```python
from build123d import *

# Parameters (mm, degrees)
SKETCH_1_R               = 3.2
EXTRUDE_1_DEPTH          = 5
CUT_EXTRUDE_1_DEPTH      = 5
CUT_EXTRUDE_1_DEPTH_BACK = 5
SKETCH_2_R               = 1.5


with BuildPart() as part:
    # Sketch 1 → Extrude 1 (new body)
    with BuildSketch(Plane.XY):
        with BuildLine():
            Line((-3.31662479, -5), (-8.660254038, -5))
            Line((-8.660254038, -5), (-8.660254038, 5))
            Line((-8.660254038, 5), (-4, 5))
            Line((-4, 5), (-4, 9.16515139))
            Line((-4, 9.16515139), (3, 9.16515139))
            Line((3, 9.16515139), (3, 5))
            Line((3, 5), (6.81662479, 5))
            Line((6.81662479, 5), (6.81662479, -5))
            Line((6.81662479, -5), (3.31662479, -5))
            ThreePointArc((3.31662479, -5), (0, -6), (-3.31662479, -5))
        make_face()
        Circle(SKETCH_1_R, mode=Mode.SUBTRACT)
    extrude(amount=EXTRUDE_1_DEPTH)

    # Sketch 2 → Cut-Extrude 1 (cut, two sides: drawn at the far end of the back side and taken through both)
    with BuildSketch(Plane.XZ.offset(5).offset(-CUT_EXTRUDE_1_DEPTH_BACK)):
        with Locations(Location((0, 2.9, 0), (0, 0, 90))):
            Circle(SKETCH_2_R)
    extrude(amount=CUT_EXTRUDE_1_DEPTH + CUT_EXTRUDE_1_DEPTH_BACK, mode=Mode.SUBTRACT)


solid = part.part
```
The listing builds one solid part. Answer for the finished solid, in the listing's coordinates (mm). A direction names the side the tool comes from. Give positions to 0.01 mm unless a question says otherwise; leave off trailing zeros. Order: outer loops, then holes, each group sorted by start corner. A loop starts at its lowest first (then second) coordinate and runs counter-clockwise, first axis right, second up. Notation, with made-up numbers: (37, 40) - (51, 40) arc R24 cw to (51, 73) - close; hole circle Ø3 at (71, 85). An arc over 180 degrees is marked (long way). Use one line per item in the form item = value. Start each with the question number.
(1) The mould has two halves that part along X. Classify faces 1 (the cylindrical face through (-0.45, -4.39, 4.33)), 2 (the flat face through (-6, -5, 2)), 3 (the flat face through (-4, 7, 2)): released by +X, released by -X, zero draft, split by the parting line, or undercut.
(2) A cutting plane is placed at D-D, the plane x = -2. Write down the section's boundary in (y, z).
(3) For faces 4 (the flat face through (-6, 5, 2)), 5 (the flat face through (5, -5, 2)), 6 (the flat face through (5, 5, 2)), determine the directions among +Z, -Z, +X, -X, +Y, -Y from which every point of the face is accessible in a straight line to the end or side of a thin tool.
(4) A cutting plane is placed at B-B, the plane x = 0. Write down the section's boundary in (y, z).
(5) Consider line 1 (X direction, y = -4.8, z = 2.9); line 2 (Y direction, x = -5, z = 1.5); line 3 (X direction, y = 5.25, z = 2.6). Determine where each line is inside the solid, lowest interval first. Write a range as from..to.
(6) Flat-ended cylindrical pins translate along their axes: pin 1 Ø3 at (x, z) = (-2.5, 1) entering from -Y; pin 2 Ø1.4 at (x, z) = (-6.5, 2) entering from +Y; pin 3 Ø1.2 at (y, z) = (7, 3.5) entering from -X. Find the tip coordinate at first contact, or state that the pin passes through.
(7) A cutting plane is placed at C-C, the plane z = 0.85. Write down the section's boundary in (x, y), then the cut area to 3 significant figures.
(8) A cutting plane is placed at A-A, the plane y = 0. Write down the section's boundary in (x, z).
Ans:
q1.face_1 = undercut
q1.face_2 = zero draft
q1.face_3 = released by -X
q2.outline = (-5.66, 0) - (-2.5, 0) - (-2.5, 5) - (-5.66, 5) - close; (2.5, 0) - (9.17, 0) - (9.17, 5) - (2.5, 5) - close
q3.face_4 = +Z, -Z, -X, +Y
q3.face_5 = +Z, -Z, +X, -Y
q3.face_6 = +Z, -Z, +X, +Y
q4.outline = (-6, 0) - (-3.2, 0) - (-3.2, 1.4) - (-6, 1.4) - close; (-6, 4.4) - (-3.2, 4.4) - (-3.2, 5) - (-6, 5) - close; (3.2, 0) - (9.17, 0) - (9.17, 5) - (3.2, 5) - close
q5.line_1 = -8.66..-1.5, 1.5..6.82
q5.line_2 = -5..5
q5.line_3 = -4..3
q6.pin_1 = -5.92
q6.pin_2 = 5
q6.pin_3 = -4
q7.outline = (-8.66, -5) - (-3.32, -5) arc R6 ccw to (3.32, -5) - (6.82, -5) - (6.82, 5) - (3, 5) - (3, 9.17) - (-4, 9.17) - (-4, 5) - (-8.66, 5) - close; hole circle Ø6.4 at (0, 0)
q7.area = 156 mm^2
q8.outline = (-8.66, 0) - (-3.2, 0) - (-3.2, 5) - (-8.66, 5) - close; (3.2, 0) - (6.82, 0) - (6.82, 5) - (3.2, 5) - close
